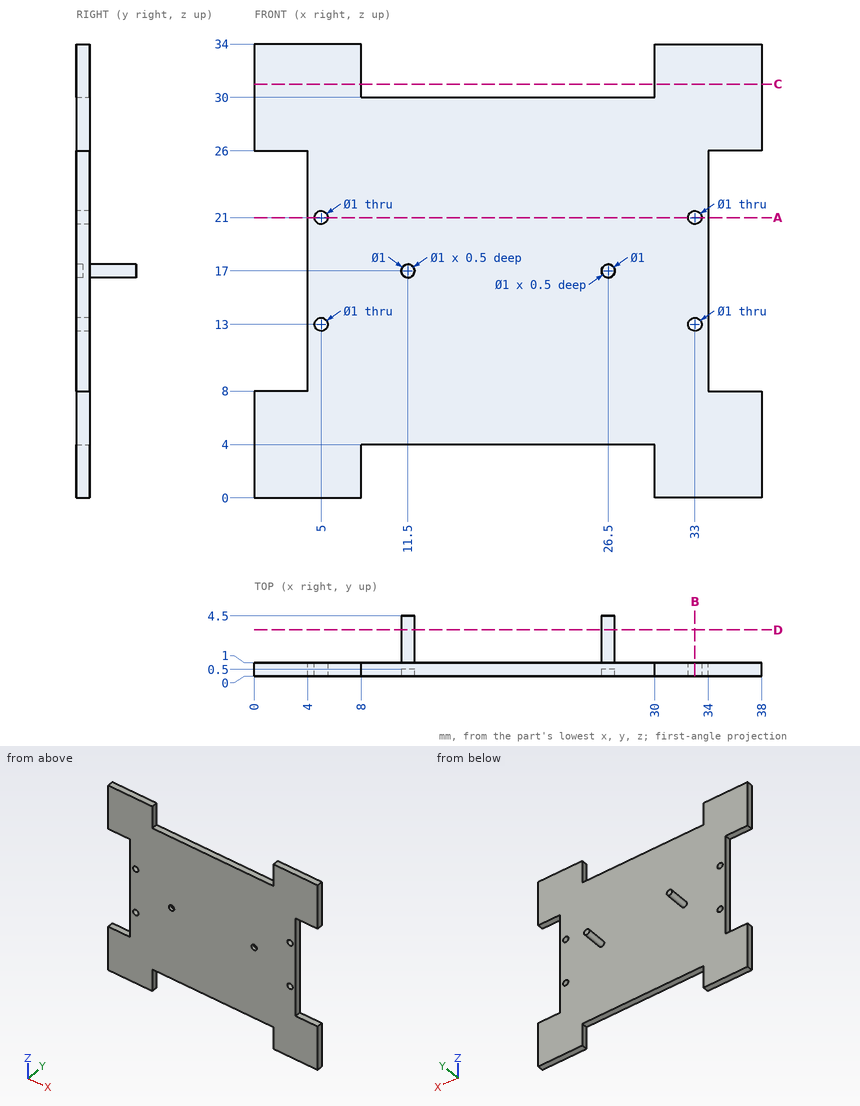
Drawing for the job (mm, zero at the part's lowest x, y, z). Round coordinates to 2 decimals unless told otherwise and drop trailing zeros. Write each loop counter-clockwise with the first axis right and the second up, starting at its lowest first coordinate (ties: lowest second). Pieces come first, ordered by that corner, then holes. Notation, with made-up numbers: (53, -14) - (94, -14) arc R17 cw to (94, -5) - close; hole circle Ø1 at (48.5, 36). An arc over 180 degrees is marked (long way). Write item = value, one per line. Start each with the question number.
Q1. Band-saw the part on C-C (z = 31). Give the cut face in (x, y).
Q2. Band-saw the part on B-B (x = 33). Give the cut face in (y, z).
Q3. Band-saw the part on A-A (z = 21). Give the cut face in (x, y).
Q4. Probe L1, parallel to Z at x = 5, y = 0.8; L2, parallel to Z at x = 26.5, y = 0.2; L3, parallel to Y at x = 3.5, z = 29. List the from-to ranges inside material, lowest first. Write a range as from..to.
Q5. Band-saw the part on D-D (y = 3.45). Give the cut face in (x, z).
Q6. Drop flat-ended pins along their axis: pin 1 (1.1 mm diameter, centred on x = 20, y = 0.5, fed in from -Z); pin 2 (0.5 mm diameter, centred on x = 11.5, z = 17, fed in from -Y); pin 3 (1.1 mm diameter, centred on x = 23, y = 0.5, fed in from +Z). Give the stop position or say it passes through.
Answers below:
q1.outline = (0, 0) - (8, 0) - (8, 1) - (0, 1) - close; (30, 0) - (38, 0) - (38, 1) - (30, 1) - close
q2.outline = (0, 0) - (1, 0) - (1, 12.5) - (0, 12.5) - close; (0, 13.5) - (1, 13.5) - (1, 20.5) - (0, 20.5) - close; (0, 21.5) - (1, 21.5) - (1, 34) - (0, 34) - close
q3.outline = (4, 0) - (4.5, 0) - (4.5, 1) - (4, 1) - close; (5.5, 0) - (32.5, 0) - (32.5, 1) - (5.5, 1) - close; (33.5, 0) - (34, 0) - (34, 1) - (33.5, 1) - close
q4.L1 = 0..12.5, 13.5..20.5, 21.5..34
q4.L2 = 4..16.5, 17.5..30
q4.L3 = 0..1
q5.outline = circle Ø1 at (11.5, 17); circle Ø1 at (26.5, 17)
q6.pin_1 = 4
q6.pin_2 = 0.5
q6.pin_3 = 30
